```python
from build123d import *

# Parameters (mm, degrees)
PAD_DEPTH    = 14
FILLET_R     = 0.29
SKETCH001_R  = 2.5
POCKET_DEPTH = 4.301


with BuildPart() as part:
    # Sketch → Pad (new body)
    with BuildSketch(Plane.XZ):
        Polygon((-2.75, 0), (2.75, 0), (2.75, -0.6), (4, -0.6), (4, -1.6), (1.75, -4.3), (-1.75, -4.3), (-4, -1.6), (-4, -0.6), (-2.75, -0.6), align=None)
    extrude(amount=PAD_DEPTH)

    # Fillet
    fillet_edges = [part.edges().sort_by_distance(p)[0] for p in [
        (1.75, -7, -4.3),
        (4, -7, -1.6),
        (4, -7, -0.6),
        (-1.75, -7, -4.3),
        (-4, -7, -1.6),
        (-4, -7, -0.6),
        (2.75, -7, -0.6),
        (2.75, -7, 0),
        (-2.75, -7, -0.6),
        (-2.75, -7, 0),
    ]]
    fillet(fillet_edges, radius=FILLET_R)

    # Sketch001 → Pocket (cut, through all)
    with BuildSketch(Plane.XY):
        with Locations((0, -10)):
            Circle(SKETCH001_R)
    extrude(amount=-POCKET_DEPTH, mode=Mode.SUBTRACT)

    # Sphere → Sphere (revolve)
    with BuildSketch(Plane(origin=(0, -4, -4), x_dir=(1, 0, 0), z_dir=(0, 0, 1))):
        with BuildLine():
            ThreePointArc((0, -1.2), (1.2, 0), (0, 1.2))
            Line((0, 1.2), (0, -1.2))
        make_face()
    revolve(axis=Axis((0, -4, -4), (0, 1, 0)))


solid = part.part
```
Can you work these out from the model? Positions are in its coordinate system, mm. A direction names the side the tool comes from. Coordinates: 2 decimals unless noted, no trailing zeros. Write each loop counter-clockwise with the first axis right and the second up, starting at its lowest first coordinate (ties: lowest second). Pieces come first, ordered by that corner, then holes. Notation, with made-up numbers: (49.5, -14) - (82.5, -14) arc R28 cw to (82.5, 22) - close; hole circle Ø2 at (5, 5). An arc over 180 degrees is marked (long way). Return JSON: item names as keys, results as strings.
Q1. On a 3-axis mill with a long thin cutter (end or side, diameter ignored), from which of +Z, -Z, +X, -X, +Y, -Y can I reach the whole of each face in a straight line? I mean faces 4 (the flat face through (0, -4, 0)), 5 (the flat face through (0, -13, -4.3)). Say none if no direction works.
Computed values:
{"face 4": "+Z, +X, -X, +Y, -Y", "face 5": "-Z, +X, -X, -Y"}
Q2. Please list where these lines run through material, in increasing order: L1, parallel to Y at x = 0, z = -1.3; L2, parallel to Z at x = -0.5, y = -1.25; L3, parallel to Z at x = 2, y = -0.75. Write a range as from..to.
Computed values:
{"L1": "y = -14..-12.5, -7.5..0", "L2": "z = -4.3..0", "L3": "z = -4..0"}
Q3. If we section it at C-C (z = -1.3): Please give me the cut outline in (x, y), then the cut area to 3 significant figures.
Computed values:
{"outline": "(-4, -14) - (4, -14) - (4, 0) - (-4, 0) - close; hole circle Ø5 at (0, -10)", "area": "92.4 mm2"}
Q4. Thinking about a two-plate mould opening in Y: for faces 1 (the cylindrical face through (-0.33, -7.52, -2.12)), 2 (the flat face through (0, -14, -2)), 3 (the flat face through (2.9, -6.9, -2.92)), which applies, +Y half, -Y half, draft (parallel to the pull), parting line (faces both ways), or undercut?
Computed values:
{"face 1": "undercut", "face 2": "-Y half", "face 3": "draft"}
Q5. I'm going to push flat-ended pins straight in: pin 1 Ø3 at (y, z) = (-2, -3.5) entering from +X; pin 2 Ø1 at (x, y) = (-0.5, -3) entering from -Z; pin 3 Ø1 at (y, z) = (-5.5, -4.5) entering from -X; pin 4 Ø3 at (x, z) = (0, -3) entering from +Y. Where does each tip first touch, or does it pass through?
Computed values:
{"pin 1": "stops at x = 3.67", "pin 2": "stops at z = -5.03", "pin 3": "stops at x = -2", "pin 4": "stops at y = 0"}
Q6. If we section it at A-A (y = -8.5): Please give me the cut outline in (x, z) (3 decimals), then the cut area to 3 significant figures.
Computed values:
{"outline": "(-4, -1.495) arc R0.29 ccw to (-3.933, -1.681) - (-2, -4) - (-2, 0) - (-2.46, 0) arc R0.29 ccw to (-2.75, -0.29) - (-2.75, -0.31) arc R0.29 cw to (-3.04, -0.6) - (-3.71, -0.6) arc R0.29 ccw to (-4, -0.89) - close; (2, -4) - (3.933, -1.681) arc R0.29 ccw to (4, -1.495) - (4, -0.89) arc R0.29 ccw to (3.71, -0.6) - (3.04, -0.6) arc R0.29 cw to (2.75, -0.31) - (2.75, -0.29) arc R0.29 ccw to (2.46, 0) - (2, 0) - close", "area": "9.66 mm2"}
Q7. If we section it at B-B (x = 0): Please give me the cut outline in (y, z).
Computed values:
{"outline": "(-14, -4.3) - (-12.5, -4.3) - (-12.5, 0) - (-14, 0) - close; (-7.5, -4.3) - (-5.16, -4.3) arc R1.2 ccw to (-2.84, -4.3) - (0, -4.3) - (0, 0) - (-7.5, 0) - close"}
Q8. If we section it at D-D (y = -1): Please give me the cut outline in (x, z) (3 decimals), then the cut area to 3 significant figures.
Computed values:
{"outline": "(-4, -1.495) arc R0.29 ccw to (-3.933, -1.681) - (-1.837, -4.196) arc R0.29 ccw to (-1.614, -4.3) - (1.614, -4.3) arc R0.29 ccw to (1.837, -4.196) - (3.933, -1.681) arc R0.29 ccw to (4, -1.495) - (4, -0.89) arc R0.29 ccw to (3.71, -0.6) - (3.04, -0.6) arc R0.29 cw to (2.75, -0.31) - (2.75, -0.29) arc R0.29 ccw to (2.46, 0) - (-2.46, 0) arc R0.29 ccw to (-2.75, -0.29) - (-2.75, -0.31) arc R0.29 cw to (-3.04, -0.6) - (-3.71, -0.6) arc R0.29 ccw to (-4, -0.89) - close", "area": "26.8 mm2"}
